Input: part model. Units: mm. Frame: model coordinates. Face numbers are marked on the shaded views. A direction names the side the tool comes from. Coordinates: 2 decimals unless noted, no trailing zeros. Loops run counter-clockwise (first coordinate to the right, second up) from the corner with the lowest first, then second, coordinate; pieces in that order, holes last. Notation, with made-up numbers: (49, 88.25) - (72, 88.25) arc R35 cw to (72, 120.25) - close; hole circle Ø4 at (66.5, 12). An arc over 180 degrees is marked (long way). Use one line per item in the form item = value.
Autodesk Inventor part; units mm, degrees
ref_plane "YZ Plane" through (0, 0, 0) normal (1, 0, 0) x (0, 1, 0)
ref_plane "XZ Plane" through (0, 0, 0) normal (0, 1, 0) x (-1, 0, 0)
ref_plane "XY Plane" through (0, 0, 0) normal (0, 0, 1) x (1, 0, 0)
sketch "Sketch1" plane through (0, 0, 0) normal (0, 1, 0) x (-1, 0, 0)
  line L0 (-17, 15) -> (17, 15)
  line L1 (17, 15) -> (17, -15)
  line L2 (17, -15) -> (-17, -15)
  line L3 (-17, -15) -> (-17, 15)
  line L4 (-17, 15) -> (17, -15) construction
  line L5 (17, 15) -> (-17, -15) construction
  line L6 (-10, 15) -> (10, 15)
  line L7 (10, 15) -> (10, -15)
  line L8 (10, -15) -> (-10, -15)
  line L9 (-10, -15) -> (-10, 15)
  line L10 (-10, 15) -> (10, -15) construction
  line L11 (10, 15) -> (-10, -15) construction
  line L12 (-2.5, 15) -> (2.5, 15)
  line L13 (2.5, 15) -> (2.5, -15)
  line L14 (2.5, -15) -> (-2.5, -15)
  line L15 (-2.5, -15) -> (-2.5, 15)
  line L16 (-2.5, 15) -> (2.5, -15) construction
  line L17 (2.5, 15) -> (-2.5, -15) construction
  point P0 (0, 0)
  point P1 (12.5, 9)
  dimension "d0" = 20
  dimension "d1" = 5
  dimension "d2" = 34
  dimension "d3" = 30
  dimension "d4" = 6
  dimension "d5" = 4.5
extrude "Extrusion1" add sketch "Sketch1" along normal blind 2 contours L0 L15 L2 L9 | L0 L7 L2 L13
extrude "Extrusion2" add sketch "Sketch1" along normal blind 7 contours L0 L9 L2 L3 | L0 L1 L2 L7
extrude "Extrusion3" add sketch "Sketch1" along normal blind 4 contours L0 L13 L2 L15
hole "Hole1" at (-12.5, 0, 9) direction (0, 1, 0) diameter 4 end through all
pattern_linear "Rectangular Pattern1" count 2 spacing 18 along (0, 0, -1) count 2 spacing 25 along (1, 0, 0) of "Hole1"
properties part number "Linear Bearing Platform Adapter Back" material "PC/ABS Plastic"
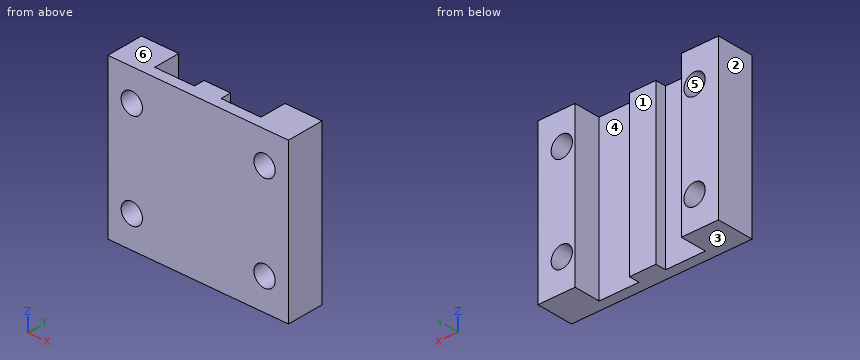
Q1. Set-up query: the marked faces 1 and 2. Return all of +Z, -Z, +X, -X, +Y, -Y with unobstructed straight access to the full face (end or side cutting, diameter ignored); none if empty.
Check values:
face_1 = +Z, -Z, +Y
face_2 = +Z, -Z, -X, +Y, -Y
Q2. Cut plane B-B, the plane z = -9. Return loops of the section in (x, y), then the cut area to 3 significant figures.
Check values:
outline = (-17, 0) - (-14.5, 0) - (-14.5, 7) - (-17, 7) - close; (-10.5, 0) - (10.5, 0) - (10.5, 7) - (10, 7) - (10, 2) - (2.5, 2) - (2.5, 4) - (-2.5, 4) - (-2.5, 2) - (-10, 2) - (-10, 7) - (-10.5, 7) - close; (14.5, 0) - (17, 0) - (17, 7) - (14.5, 7) - close
area = 92.0 mm²
Q3. Ray query, line 1 along Z through (x, y) = (-12.5, 5); line 2 along X through (y, z) = (2.75, -2); line 3 along X through (y, z) = (3.5, 9). Return the intervals inside material, ascending. Write a range as [from, to].
Check values:
line_1 = [-15, -11], [-7, 7], [11, 15]
line_2 = [-17, -10], [-2.5, 2.5], [10, 17]
line_3 = [-17, -14.5], [-10.5, -10], [-2.5, 2.5], [10, 10.5], [14.5, 17]
Q4. Cut plane A-A, the plane y = 3. Return loops of the section in (x, z).
Check values:
outline = (-17, -15) - (-10, -15) - (-10, 15) - (-17, 15) - close; (-2.5, -15) - (2.5, -15) - (2.5, 15) - (-2.5, 15) - close; (10, -15) - (17, -15) - (17, 15) - (10, 15) - close; hole circle Ø4 at (-12.5, -9); hole circle Ø4 at (-12.5, 9); hole circle Ø4 at (12.5, -9); hole circle Ø4 at (12.5, 9)
Q5. Cut plane D-D, the plane y = 6.25. Return loops of the section in (x, z).
Check values:
outline = (-17, -15) - (-10, -15) - (-10, 15) - (-17, 15) - close; (10, -15) - (17, -15) - (17, 15) - (10, 15) - close; hole circle Ø4 at (-12.5, -9); hole circle Ø4 at (-12.5, 9); hole circle Ø4 at (12.5, -9); hole circle Ø4 at (12.5, 9)
Q6. Pull-direction query (Z, two-part tool) for the marked faces 3, 4, 5 and 6; classes: pulls with the +Z half, pulls with the -Z half, needs draft (parallel to the pull), parting line crosses it, or undercut.
Check values:
face_3 = pulls with the -Z half
face_4 = needs draft
face_5 = undercut
face_6 = pulls with the +Z half
Q7. Cut plane C-C, the plane x = 12.5. Return loops of the section in (y, z), then the cut area to 3 significant figures.
Check values:
outline = (0, -15) - (7, -15) - (7, -11) - (0, -11) - close; (0, -7) - (7, -7) - (7, 7) - (0, 7) - close; (0, 11) - (7, 11) - (7, 15) - (0, 15) - close
area = 154 mm²
Q8. First-contact query: P1, Ø2, axis at x = 2, z = 9, coming from the +Y side; P2, Ø4, axis at x = -5.5, z = -4.5, coming from the +Y side. Flat tips, straight axial feed; report the tip coordinate or a pass-through.
Check values:
P1 = 4
P2 = 2
